Check sheet for the modelled part. Datum: model origin and axes. Units: mm. Coordinates: 2 decimals unless noted, no trailing zeros. Write each loop counter-clockwise with the first axis right and the second up, starting at its lowest first coordinate (ties: lowest second). Pieces come first, ordered by that corner, then holes. Notation, with made-up numbers: (65.25, -2.5) -> (119.25, -2.5) arc R15 cw to (119.25, 3.5) -> close; hole circle Ø10 at (34, 87). An arc over 180 degrees is marked (long way). Put each result on its own line as item: value.
```python
from build123d import *

# Parameters (mm, degrees)
BOSS_EXTRUDE1_DEPTH = 1.5875


with BuildPart() as part:
    # Sketch1 → Boss-Extrude1 (new body, symmetric)
    with BuildSketch(Plane(origin=(0, 0, 0), x_dir=(1, 0, 0), z_dir=(0, 1, 0))):
        Polygon((222.25, 41.544875), (-228.6, 41.544875), (-228.6, 8.73125), (-222.25, 8.73125), (-203.2, 8.73125), (-203.2, 5.55625), (-222.25, 5.55625), (-228.6, 5.55625), (-228.6, -5.55625), (-222.25, -5.55625), (-203.2, -5.55625), (-203.2, -8.73125), (-222.25, -8.73125), (-228.6, -8.73125), (-228.6, -41.544875), (222.25, -41.544875), (222.25, -48.021875), (-228.6, -48.021875), (-228.6, -58.7375), (190.5, -58.7375), (228.6, -58.7375), (228.6, -8.73125), (222.25, -8.73125), (203.2, -8.73125), (203.2, -5.55625), (222.25, -5.55625), (228.6, -5.55625), (228.6, 5.55625), (222.25, 5.55625), (203.2, 5.55625), (203.2, 8.73125), (222.25, 8.73125), (228.6, 8.73125), (228.6, 58.7375), (190.5, 58.7375), (-228.6, 58.7375), (-228.6, 48.021875), (222.25, 48.021875), align=None)
        Polygon((222.25, 35.194875), (222.25, 15.875), (196.85, 15.875), (196.85, -15.875), (222.25, -15.875), (222.25, -35.194875), (-222.25, -35.194875), (-222.25, -15.875), (-196.85, -15.875), (-196.85, 15.875), (-222.25, 15.875), (-222.25, 35.194875), align=None, mode=Mode.SUBTRACT)
    extrude(amount=BOSS_EXTRUDE1_DEPTH, both=True)


solid = part.part
```
Q1. Cross-section at B-B (x = 30.5). Record the cut outline in (y, z).
Recorded:
outline: (-1.59, -58.74) -> (1.59, -58.74) -> (1.59, -48.02) -> (-1.59, -48.02) -> close; (-1.59, -41.54) -> (1.59, -41.54) -> (1.59, -35.19) -> (-1.59, -35.19) -> close; (-1.59, 35.19) -> (1.59, 35.19) -> (1.59, 41.54) -> (-1.59, 41.54) -> close; (-1.59, 48.02) -> (1.59, 48.02) -> (1.59, 58.74) -> (-1.59, 58.74) -> close
Q2. Material ranges on line 1 along Z through (x, y) = (162.5, -0.2); line 2 along Z through (x, y) = (201.5, 1.35) (1 decimal); line 3 along X through (y, z) = (-1, 2), recorded low to high.
Recorded:
line 1: z = -58.74 to -48.02, -41.54 to -35.19, 35.19 to 41.54, 48.02 to 58.74
line 2: z = -58.7 to -48, -41.5 to -35.2, -15.9 to 15.9, 35.2 to 41.5, 48 to 58.7
line 3: x = -228.6 to -196.85, 196.85 to 228.6
Q3. Depth check by flat-ended pin: P1, Ø6, axis at x = -8, z = 30, coming from the -Y side; P2, Ø1.6, axis at y = 0.5, z = -46, coming from the -X side. Enter the tip coordinate at first touch or a pass-through.
Recorded:
P1: passes through
P2: stops at x = 222.25
Q4. Cross-section at A-A (z = 0.5). Record the cut outline in (x, y).
Recorded:
outline: (-228.6, -1.59) -> (-196.85, -1.59) -> (-196.85, 1.59) -> (-228.6, 1.59) -> close; (196.85, -1.59) -> (228.6, -1.59) -> (228.6, 1.59) -> (196.85, 1.59) -> close
Q5. Cross-section at C-C (z = -26.5). Record the cut outline in (x, y).
Recorded:
outline: (-228.6, -1.59) -> (-222.25, -1.59) -> (-222.25, 1.59) -> (-228.6, 1.59) -> close; (222.25, -1.59) -> (228.6, -1.59) -> (228.6, 1.59) -> (222.25, 1.59) -> close
